from build123d import *

# Parameters (mm, degrees)
F0_W      = 203.2
F0_H      = 254
F1_DEPTH  = 7.62
F2_W      = 101.6
F2_H      = 76.2
F3_DEPTH  = 88.9
F4_R      = 4.064
F5_DEPTH  = 88.9
F8_DEPTH  = 101.6
F10_DEPTH = 30.48


with BuildPart() as f1:
    # F0 (on Top) → F1 (new body)
    with BuildSketch(Plane.XY):
        with Locations((0, -25.4)):
            Rectangle(F0_W, F0_H)
    extrude(amount=F1_DEPTH)

    # F2 (on face) → F3 (join)
    with BuildSketch(Plane.XY.offset(7.62)):
        Rectangle(F2_W, F2_H)
    extrude(amount=F3_DEPTH)

    # F4 (on face) → F5 (cut)
    with BuildSketch(Plane.XY.offset(96.52)):
        with Locations((0, 25.4)):
            Circle(F4_R)
    extrude(amount=-F5_DEPTH, mode=Mode.SUBTRACT)

    # F6 (on face) → F7 (revolve, cut)
    with BuildSketch(Plane.XY.offset(96.52)):
        with BuildLine():
            ThreePointArc((0, -29.464), (2.8736819587, -28.2736819587), (4.064, -25.4))
            Line((4.064, -25.4), (4.064, 25.4))
            ThreePointArc((4.064, 25.4), (2.8736819587, 22.5263180413), (0, 21.336))
            Line((0, 21.336), (0, -29.464))
        make_face()
    revolve(axis=Axis((0, 0, 96.52), (0, -1, 0)), mode=Mode.SUBTRACT)

    # F8 (add): a face of the model
    f8_faces = [f1.faces().sort_by_distance(p)[0] for p in [
        (0, -38.1, 52.07),
    ]]
    extrude(f8_faces, amount=F8_DEPTH)

    # F9 (on face) → F10 (cut)
    with BuildSketch(Plane.XY.offset(96.52)):
        with BuildLine():
            Line((-3.175, -81.915), (-3.175, -88.6484904355))
            ThreePointArc((-3.175, -88.6484904355), (0, -114.935), (3.175, -88.6484904355))
            Line((3.175, -88.6484904355), (3.175, -81.915))
            Line((3.175, -81.915), (-3.175, -81.915))
        make_face()
    extrude(amount=-F10_DEPTH, mode=Mode.SUBTRACT)


solid = f1.part
Could you check a few things on this model? Use its own coordinates, in mm. A direction names the side the tool comes from. Coordinates: 2 decimals unless noted, no trailing zeros. Order: outer loops, then holes, each group sorted by start corner. A loop starts at its lowest first (then second) coordinate and runs counter-clockwise, first axis right, second up. Notation, with made-up numbers: (62, -35) - (72, -35) arc R14 cw to (72, -27) - close; hole circle Ø9 at (36.5, -9.5). An arc over 180 degrees is marked (long way). Answer in a Markdown table with one row per item. Add a question column.
(1) Will these pins go through, and if not, where does the flat tip stop? pin 1 (6 mm diameter, centred on y = 11, z = 79.5, fed in from +X); pin 2 (1.5 mm diameter, centred on x = 37.5, z = 44, fed in from -Y); pin 3 (3 mm diameter, centred on x = -59, y = 40, fed in from +Z).
(2) If we mould it in two halves opening along Y, with no side actions, what happens to faces 1 (the face through (-1, -139.7, 51)), 2 (the face through (-1, 61, 7.62)), 3 (the face through (-0.881, 21.433, 52.692))? For each: released by +Y, released by -Y, zero draft, split by the parting line, or undercut.
(3) I need wall thicknesses on L1, parallel to X at y = 25, z = 58; L2, parallel to Y at x = 0, z = 45; L3, parallel to X at y = -86.5, z = 73.5 (3 decimals). Which ranges of each line are inside material? Lowest first, please.
(4) If we section it at B-B, the plane y = -101.6: Please give me the cut outline in (x, z) (3 decimals).
(5) If we section it at C-C, the plane x = 0: Please give me the cut outline in (y, z) (3 decimals).
(6) If we section it at D-D, the plane x = -26.5: Please give me the cut outline in (y, z).
(7) If we section it at A-A, the plane z = 58: Please give me the cut outline in (x, y).
(8) On a 3-axis mill with a long thin cutter (end or side, diameter ignored), from which of +Z, -Z, +X, -X, +Y, -Y can I reach the whole of each face in a straight line? I mean faces 4 (the face through (-50.8, -50, 51)), 5 (the face through (-1, 38.1, 51)), 6 (the face through (-3.175, -85, 81)), 7 (the face through (50.8, -50, 51)). Say none if no direction works.
Results are:
| question | item | result |
|---|---|---|
| 1 | pin 1 | stops at x = 50.8 |
| 1 | pin 2 | stops at y = -139.7 |
| 1 | pin 3 | stops at z = 7.62 |
| 2 | face 1 | released by -Y |
| 2 | face 2 | zero draft |
| 2 | face 3 | undercut |
| 3 | L1 | x = -50.8 to -4.04, 4.04 to 50.8 |
| 3 | L2 | y = -139.7 to 21.34, 29.46 to 38.1 |
| 3 | L3 | x = -50.8 to -3.175, 3.175 to 50.8 |
| 4 | outline | (-101.6, 0) - (101.6, 0) - (101.6, 7.62) - (50.8, 7.62) - (50.8, 96.52) - (13.335, 96.52) - (13.335, 66.04) - (-13.335, 66.04) - (-13.335, 96.52) - (-50.8, 96.52) - (-50.8, 7.62) - (-101.6, 7.62) - close |
| 5 | outline | (-152.4, 0) - (101.6, 0) - (101.6, 7.62) - (38.1, 7.62) - (38.1, 96.52) - (29.464, 96.52) - (29.464, 7.62) - (21.336, 7.62) - (21.336, 92.456) - (-25.4, 92.456) arc R4.064 cw to (-29.464, 96.52) - (-81.915, 96.52) - (-81.915, 66.04) - (-114.935, 66.04) - (-114.935, 96.52) - (-139.7, 96.52) - (-139.7, 7.62) - (-152.4, 7.62) - close |
| 6 | outline | (-152.4, 0) - (101.6, 0) - (101.6, 7.62) - (38.1, 7.62) - (38.1, 96.52) - (-139.7, 96.52) - (-139.7, 7.62) - (-152.4, 7.62) - close |
| 7 | outline | (-50.8, -139.7) - (50.8, -139.7) - (50.8, 38.1) - (-50.8, 38.1) - close; hole circle Ø8.13 at (0, 25.4) |
| 8 | face 4 | +Z, -X, +Y, -Y |
| 8 | face 5 | +Z, +X, -X, +Y |
| 8 | face 6 | +Z |
| 8 | face 7 | +Z, +X, +Y, -Y |
